Here's how the part is built. I have some questions about the finished solid (model axes, mm). Face numbers are marked on the shaded views. A direction names the side the tool comes from. Round coordinates to 2 decimals unless told otherwise and drop trailing zeros. Write each loop counter-clockwise with the first axis right and the second up, starting at its lowest first coordinate (ties: lowest second). Pieces come first, ordered by that corner, then holes. Notation, with made-up numbers: (-7.75, 47.5) - (1.25, 47.5) arc R17 cw to (1.25, 80.5) - close; hole circle Ø1 at (75.5, -30.5). An arc over 180 degrees is marked (long way). Write item = value, one per line. Start each with the question number.
Item 1: If I drill on line 1 along Y through (x, z) = (26, 7.5); line 2 along X through (y, z) = (-26.5, 5.75); line 3 along Y through (x, z) = (4.5, 1), over which ranges is the centre line in solid material (lowest first)? Write a range as [from, to].
Item 2: Which directions (+Z, -Z, +X, -X, +Y, -Y) give clear straight access to the entire face, cutting with the end or side of a thin tool? Please do the marked faces 5 and 6.
Item 3: Thinking about a two-plate mould opening in X: for the marked faces 1, 2, 3 and 4, which applies, pulls with the +X half, pulls with the -X half, needs draft (parallel to the pull), parting line crosses it, or undercut?
Item 4: If we section it at C-C (z = 3): Please give me the cut outline in (x, y), and give its area (3 significant figures).
Item 5: If we section it at A-A (y = -26.5): Please give me the cut outline in (x, z), and give its area (3 significant figures).
Item 6: If we section it at B-B (x = 5): Please give me the cut outline in (y, z).
Item 7: For P1, Ø1, axis at x = 11.5, z = 6.5, coming from the -Y side; P2, Ø6, axis at x = 20, z = 9, coming from the -Y side, each with a flat end and sliding along its axis, tell me the tip position at first contact or that it passes through.
```python
from build123d import *

# Parameters (mm, degrees)
EXTRUDE_1_OUTLINE_R = 1.6
EXTRUDE_1_DEPTH     = 10
CUT_EXTRUDE_2_DEPTH = 10


# Read off the part's stored shape, not the designer's step: 凸台-拉伸1
with BuildPart() as part:
    # 凸台-拉伸1 outline → 凸台-拉伸1 (new body)
    with BuildSketch(Plane.XY):
        with BuildLine():
            Line((31.599493043, -25.854101966), (38.776412907, -3.765813851))
            ThreePointArc((38.776412907, -3.765813851), (39.692208515, 0.048749382), (40, 3.959611008))
            Line((40, 3.959611008), (40, 4))
            ThreePointArc((40, 4), (38.242640687, 8.242640687), (34, 10))
            Line((34, 10), (6, 10))
            ThreePointArc((6, 10), (1.757359313, 8.242640687), (0, 4))
            ThreePointArc((0, 4), (0.622521006, 0.200308091), (2.416373879, -3.206636444))
            Line((2.416373879, -3.206636444), (20.806298091, -27.610890139))
            ThreePointArc((20.806298091, -27.610890139), (22.920924272, -29.36960617), (25.598111151, -30))
            Line((25.598111151, -30), (25.893153945, -30))
            ThreePointArc((25.893153945, -30), (29.419865459, -28.854101966), (31.599493043, -25.854101966))
        make_face()
        with Locations((26, -25.992428083)):
            Circle(EXTRUDE_1_OUTLINE_R, mode=Mode.SUBTRACT)
        with Locations((5, 4.007571917)):
            Circle(EXTRUDE_1_OUTLINE_R, mode=Mode.SUBTRACT)
        with Locations((35, 4.007571917)):
            Circle(EXTRUDE_1_OUTLINE_R, mode=Mode.SUBTRACT)
    extrude(amount=EXTRUDE_1_DEPTH)

    # 草图3 → 切除-拉伸2 (cut)
    with BuildSketch(Plane.XY.offset(10)):
        with BuildLine():
            ThreePointArc((8.419814245, -1.203630046), (8.227216542, 0.892395626), (10.017085265, 2))
            Line((10.017085265, 2), (31.252942008, 2))
            ThreePointArc((31.252942008, 2), (32.870975997, 1.175570505), (33.15505504, -0.618033989))
            Line((33.15505504, -0.618033989), (26.757172713, -20.3086911))
            ThreePointArc((26.757172713, -20.3086911), (25.185154892, -21.663228314), (23.25778866, -20.894287158))
            Line((23.25778866, -20.894287158), (8.419814245, -1.203630046))
        make_face()
    extrude(amount=-CUT_EXTRUDE_2_DEPTH, mode=Mode.SUBTRACT)


solid = part.part
```
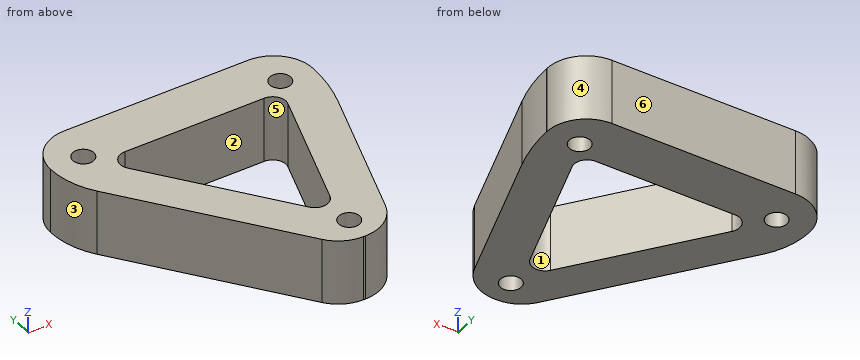
Reply:
q1.line_1 = [-30, -27.59], [-24.39, -21.33], [2, 10]
q1.line_2 = [19.97, 24.48], [27.52, 31.35]
q1.line_3 = [-5.97, 2.49], [5.53, 9.81]
q2.face_5 = +Z, -Z
q2.face_6 = +Z, -Z, +X, -X, +Y
q3.face_1 = undercut
q3.face_2 = undercut
q3.face_3 = pulls with the -X half
q3.face_4 = pulls with the +X half
q4.outline = (0, 4) arc R12 ccw to (2.42, -3.21) - (20.81, -27.61) arc R6 ccw to (25.6, -30) - (25.89, -30) arc R6 ccw to (31.6, -25.85) - (38.78, -3.77) arc R25 ccw to (40, 3.96) - (40, 4) arc R6 ccw to (34, 10) - (6, 10) arc R6 ccw to start; hole circle Ø3.2 at (5, 4.01); hole (8.42, -1.2) - (23.26, -20.89) arc R2 ccw to (26.76, -20.31) - (33.16, -0.62) arc R2 ccw to (31.25, 2) - (10.02, 2) arc R2 ccw to start; hole circle Ø3.2 at (26, -25.99); hole circle Ø3.2 at (35, 4.01)
q4.area = 713 mm2
q5.outline = (19.97, 0) - (24.48, 0) - (24.48, 10) - (19.97, 10) - close; (27.52, 0) - (31.35, 0) - (31.35, 10) - (27.52, 10) - close
q5.area = 83.4 mm2
q6.outline = (-6.64, 0) - (2.41, 0) - (2.41, 10) - (-6.64, 10) - close; (5.61, 0) - (9.92, 0) - (9.92, 10) - (5.61, 10) - close
q7.P1 = -15.92
q7.P2 = -29.41
